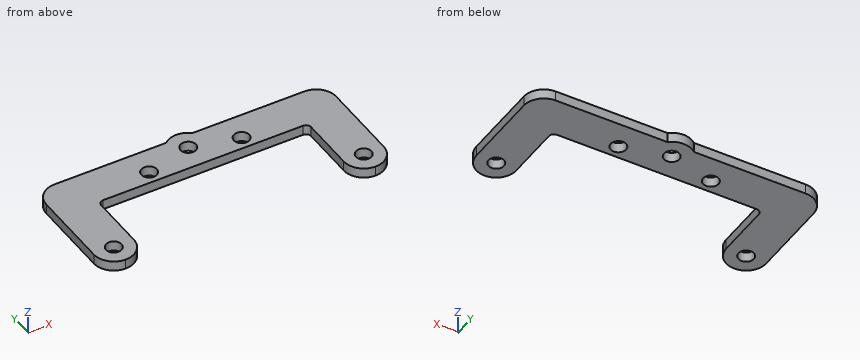
```python
from build123d import *

# Parameters (mm, degrees)
F0_R     = 1.55
F1_DEPTH = 2


with BuildPart() as f1:
    # F0 (on Top) → F1 (new body)
    with BuildSketch(Plane.XY):
        with BuildLine():
            Line((-20, -5), (20, -5))
            ThreePointArc((20, -5), (20.707107, -5.292893), (21, -6))
            Line((21, -6), (21, -17))
            ThreePointArc((21, -17), (22.171573, -19.828427), (25, -21))
            ThreePointArc((25, -21), (27.828427, -19.828427), (29, -17))
            Line((29, -17), (29, -1))
            ThreePointArc((29, -1), (27.828427, 1.828427), (25, 3))
            Line((25, 3), (2.645751, 3))
            ThreePointArc((2.645751, 3), (0, 4), (-2.645751, 3))
            Line((-2.645751, 3), (-25, 3))
            ThreePointArc((-25, 3), (-27.828427, 1.828427), (-29, -1))
            Line((-29, -1), (-29, -17))
            ThreePointArc((-29, -17), (-27.828427, -19.828427), (-25, -21))
            ThreePointArc((-25, -21), (-22.171573, -19.828427), (-21, -17))
            Line((-21, -17), (-21, -6))
            ThreePointArc((-21, -6), (-20.707107, -5.292893), (-20, -5))
        make_face()
        with Locations((-25, -17)):
            Circle(F0_R, mode=Mode.SUBTRACT)
        with Locations((25, -17)):
            Circle(F0_R, mode=Mode.SUBTRACT)
        with Locations((-9.25, -2.4)):
            Circle(F0_R, mode=Mode.SUBTRACT)
        with Locations((9.25, -2.4)):
            Circle(F0_R, mode=Mode.SUBTRACT)
        Circle(F0_R, mode=Mode.SUBTRACT)
    extrude(amount=F1_DEPTH)


solid = f1.part
```
CAD build for the part. Positions are in the model's coordinates, mm. Round coordinates to 2 decimals unless told otherwise and drop trailing zeros. Order: outer loops, then holes, each group sorted by start corner. A loop starts at its lowest first (then second) coordinate and runs counter-clockwise, first axis right, second up. Notation, with made-up numbers: (-13, 13) - (11, 13) arc R15 ccw to (11, 38) - close; hole circle Ø10 at (-39.5, 76.5). An arc over 180 degrees is marked (long way). Use CSV: the item, a comma, the result in double quotes. Start each with the question number.
1) Pin check, flat tips, straight feed: pin 1 Ø0.6 at (x, z) = (-9, 1) entering from -Y; pin 2 Ø10 at (x, y) = (5, -7) entering from -Z. Stop position of each tip, or through.
2) Saw through at D-D (z = 1.4). List the corners of the cut face in (x, y).
3) Wall check: L1, parallel to X at y = -2.5, z = 0.15; L2, parallel to Y at x = 0, z = 0.95; L3, parallel to X at y = -9, z = 0.8. Give the ranges that are in metal, low to high. Write a range as [from, to].
4) Saw through at A-A (y = -10.5). List the corners of the cut face in (x, z), and give its area (3 significant figures).
5) Saw through at B-B (x = -9.25). List the corners of the cut face in (y, z), and give its area (3 significant figures).
6) Saw through at C-C (y = -2.4). List the corners of the cut face in (x, z), and give its area (3 significant figures).
Values follow:
1,pin 1,"stops at y = -5"
1,pin 2,"stops at z = 0"
2,outline,"(-29, -17) arc R4 ccw to (-21, -17) - (-21, -6) arc R1 cw to (-20, -5) - (20, -5) arc R1 cw to (21, -6) - (21, -17) arc R4 ccw to (29, -17) - (29, -1) arc R4 ccw to (25, 3) - (2.65, 3) arc R4 ccw to (-2.65, 3) - (-25, 3) arc R4 ccw to (-29, -1) - close; hole circle Ø3.1 at (-25, -17); hole circle Ø3.1 at (-9.25, -2.4); hole circle Ø3.1 at (0, 0); hole circle Ø3.1 at (9.25, -2.4); hole circle Ø3.1 at (25, -17)"
3,L1,"x = [-29, -10.8], [-7.7, 7.7], [10.8, 29]"
3,L2,"y = [-5, -1.55], [1.55, 4]"
3,L3,"x = [-29, -21], [21, 29]"
4,outline,"(-29, 0) - (-21, 0) - (-21, 2) - (-29, 2) - close; (21, 0) - (29, 0) - (29, 2) - (21, 2) - close"
4,area,"32.0 mm2"
5,outline,"(-5, 0) - (-3.95, 0) - (-3.95, 2) - (-5, 2) - close; (-0.85, 0) - (3, 0) - (3, 2) - (-0.85, 2) - close"
5,area,"9.80 mm2"
6,outline,"(-29, 0) - (-10.8, 0) - (-10.8, 2) - (-29, 2) - close; (-7.7, 0) - (7.7, 0) - (7.7, 2) - (-7.7, 2) - close; (10.8, 0) - (29, 0) - (29, 2) - (10.8, 2) - close"
6,area,"104 mm2"
